from build123d import *

# Parameters (mm, degrees)
AUFSATZ_LINEAR_AUSTRAGEN1_DEPTH = 10
SKIZZE2_R                       = 1.6
SCHNITT_LINEAR_AUSTRAGEN1_DEPTH = 21
SKIZZE3_R                       = 3
SCHNITT_LINEAR_AUSTRAGEN2_DEPTH = 13


with BuildPart() as part:
    # Skizze1 → Aufsatz-Linear austragen1 (new body)
    with BuildSketch(Plane(origin=(0, 0, 0), x_dir=(1, 0, 0), z_dir=(0, 1, 0))):
        with BuildLine():
            Line((14, -1), (24, -1))
            Line((24, -1), (24, 19))
            Line((24, 19), (-24, 19))
            Line((-24, 19), (-24, -1))
            Line((-24, -1), (-14, -1))
            ThreePointArc((-14, -1), (0, 13), (14, -1))
        make_face()
    extrude(amount=AUFSATZ_LINEAR_AUSTRAGEN1_DEPTH)

    # Skizze2 → Schnitt-Linear austragen1 (cut, through all)
    with BuildSketch(Plane.XY.offset(1)):
        with Locations((-19, 5)):
            Circle(SKIZZE2_R)
        with Locations((19, 5)):
            Circle(SKIZZE2_R)
    extrude(amount=-SCHNITT_LINEAR_AUSTRAGEN1_DEPTH, mode=Mode.SUBTRACT)

    # Skizze3 → Schnitt-Linear austragen2 (cut)
    with BuildSketch(Plane(origin=(0, 0, -19), x_dir=(-1, 0, 0), z_dir=(0, 0, -1))):
        with Locations((-19, 5)):
            Circle(SKIZZE3_R)
        with Locations((19, 5)):
            Circle(SKIZZE3_R)
    extrude(amount=-SCHNITT_LINEAR_AUSTRAGEN2_DEPTH, mode=Mode.SUBTRACT)


solid = part.part
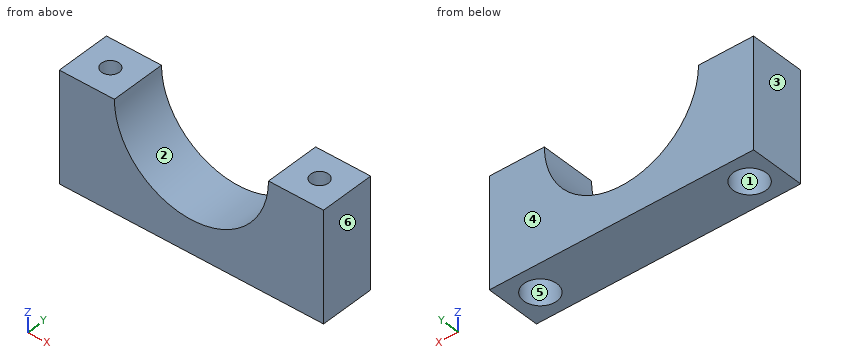
The listing builds one solid part. Answer for the finished solid, in the listing's coordinates (mm). Face numbers are marked on the shaded views. A direction names the side the tool comes from. Coordinates: 2 decimals unless noted, no trailing zeros. Order: outer loops, then holes, each group sorted by start corner. A loop starts at its lowest first (then second) coordinate and runs counter-clockwise, first axis right, second up. Notation, with made-up numbers: (44, 54) -> (74, 54) arc R27 cw to (74, 91) -> close; hole circle Ø6 at (-36.5, 55). An arc over 180 degrees is marked (long way). Answer in a Markdown table with one row per item. Add a question column.
Item 1: Find the intervals of material crossed by L1, parallel to X at y = 4, z = -0.25; L2, parallel to Y at x = 19, z = -4.25; L3, parallel to X at y = 6.25, z = -11.75, in increasing order. Write a range as from..to.
Item 2: Find section C-C (x = -19). Write down the section's boundary in (y, z).
Item 3: Find section D-D (z = -15.75). Write down the section's boundary in (x, y).
Item 4: Find section A-A (z = -0.75). Write down the section's boundary in (x, y).
Item 5: Which of the six approach directions +Z, -Z, +X, -X, +Y, -Y give full straight-line access (tool end or side, diameter ignored) to the marked faces 5 and 6?
Item 6: Find section B-B (y = 5). Write down the section's boundary in (x, z).
Item 7: Each of these flat-tipped pins is pushed along its axis until it touches: P1, Ø1, axis at x = -15, z = -4, coming from the -Y side; P2, Ø1.5, axis at x = -8.5, y = 8.5, coming from the +Z side; P3, Ø3, axis at x = -1.5, y = 3, coming from the +Z side. Where does it stop, or does it pass through?
Item 8: Determine the mould class of the marked faces 1, 2, 3 and 4 for opening direction X: +X half, -X half, draft (parallel to the pull), parting line (faces both ways), or undercut.
Result set:
| question | item | result |
|---|---|---|
| 1 | L1 | x = -24..-20.25, -17.75..-13.94, 13.94..17.75, 20.25..24 |
| 1 | L2 | y = 0..3.4, 6.6..10 |
| 1 | L3 | x = -24..-21.73, -16.27..-5.78, 5.78..16.27, 21.73..24 |
| 2 | outline | (0, -19) -> (2, -19) -> (2, -6) -> (3.4, -6) -> (3.4, 1) -> (0, 1) -> close; (6.6, -6) -> (8, -6) -> (8, -19) -> (10, -19) -> (10, 1) -> (6.6, 1) -> close |
| 3 | outline | (-24, 0) -> (24, 0) -> (24, 10) -> (-24, 10) -> close; hole circle Ø6 at (-19, 5); hole circle Ø6 at (19, 5) |
| 4 | outline | (-24, 0) -> (-13.89, 0) -> (-13.89, 10) -> (-24, 10) -> close; (13.89, 0) -> (24, 0) -> (24, 10) -> (13.89, 10) -> close; hole circle Ø3.2 at (-19, 5); hole circle Ø3.2 at (19, 5) |
| 5 | face 5 | -Z |
| 5 | face 6 | +Z, -Z, +X, +Y, -Y |
| 6 | outline | (-24, -19) -> (-22, -19) -> (-22, -6) -> (-20.6, -6) -> (-20.6, 1) -> (-24, 1) -> close; (-17.4, -6) -> (-16, -6) -> (-16, -19) -> (16, -19) -> (16, -6) -> (17.4, -6) -> (17.4, 1) -> (14, 1) arc R14 cw to (-14, 1) -> (-17.4, 1) -> close; (20.6, -6) -> (22, -6) -> (22, -19) -> (24, -19) -> (24, 1) -> (20.6, 1) -> close |
| 7 | P1 | stops at y = 0 |
| 7 | P2 | stops at z = -9.51 |
| 7 | P3 | stops at z = -12.67 |
| 8 | face 1 | undercut |
| 8 | face 2 | undercut |
| 8 | face 3 | -X half |
| 8 | face 4 | draft |
